Geometry check sheet. Reference: drawing and pictorial views, mm from the part's lowest x, y, z. Round coordinates to 2 decimals unless told otherwise and drop trailing zeros. Order: outer loops, then holes, each group sorted by start corner. A loop starts at its lowest first (then second) coordinate and runs counter-clockwise, first axis right, second up.
Q1. Cross-section at C-C on z = 2.15. Give the number of separate pieces and of enclosed holes in the cut face, then the cut area to 3 significant figures.
Q2. Cross-section at D-D on y = 17. Record the cut outline in (x, z).
Q3. Cross-section at A-A on y = 59.15. Record the cut outline in (x, z), then the cut area to 3 significant figures.
Q4. Cross-section at B-B on x = 31. Record the cut outline in (y, z).
Q5. Scan lines: probe 1 along Y at (x, z) = (62.2, 1.25); probe 2 along Y at (x, z) = (17, 0.2); probe 3 along X at (y, z) = (139.15, 1.75). Record each from-to range of solid material in increasing order.
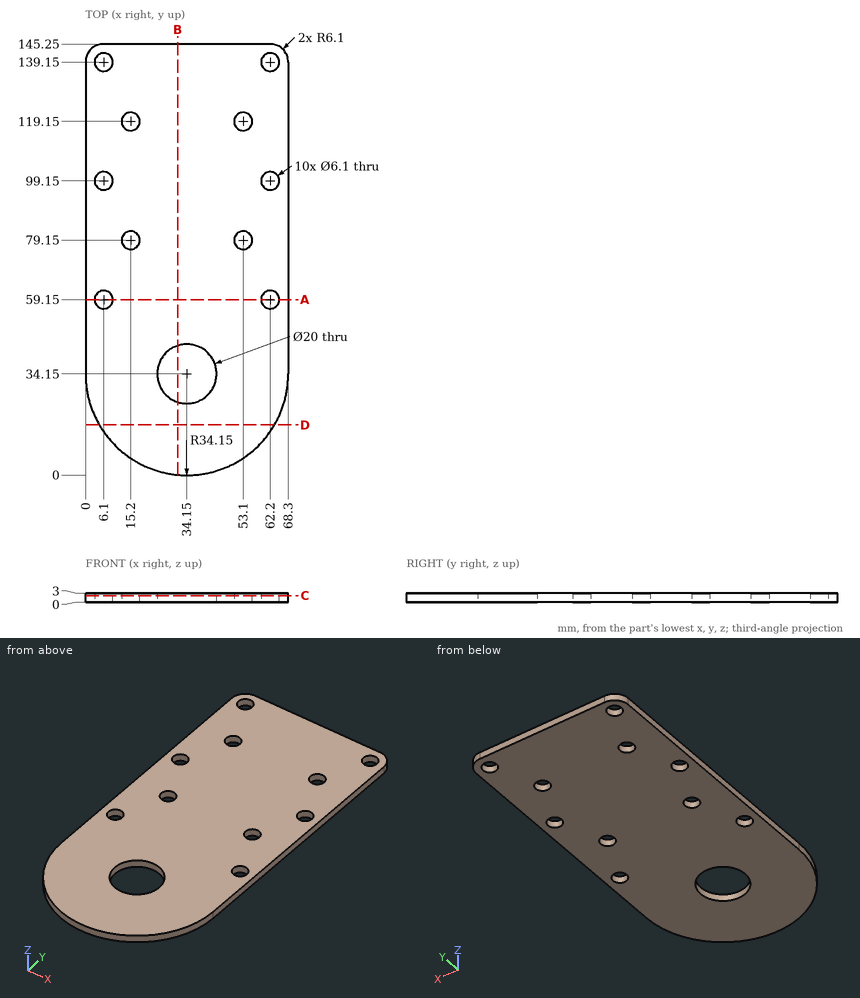
Results found:
1. separate pieces: 1
1. enclosed holes: 11
1. area: 8,800 mm2
2. outline: (4.62, 0) - (63.68, 0) - (63.68, 3) - (4.62, 3) - close
3. outline: (0, 0) - (3.05, 0) - (3.05, 3) - (0, 3) - close; (9.15, 0) - (59.15, 0) - (59.15, 3) - (9.15, 3) - close; (65.25, 0) - (68.3, 0) - (68.3, 3) - (65.25, 3) - close
3. area: 168 mm2
4. outline: (0.15, 0) - (24.66, 0) - (24.66, 3) - (0.15, 3) - close; (43.64, 0) - (145.25, 0) - (145.25, 3) - (43.64, 3) - close
5. probe 1: y = 14.67 to 56.1, 62.2 to 96.1, 102.2 to 136.1, 142.2 to 145.25
5. probe 2: y = 4.62 to 76.69, 81.61 to 116.69, 121.61 to 145.25
5. probe 3: x = 0 to 3.05, 9.15 to 59.15, 65.25 to 68.3
